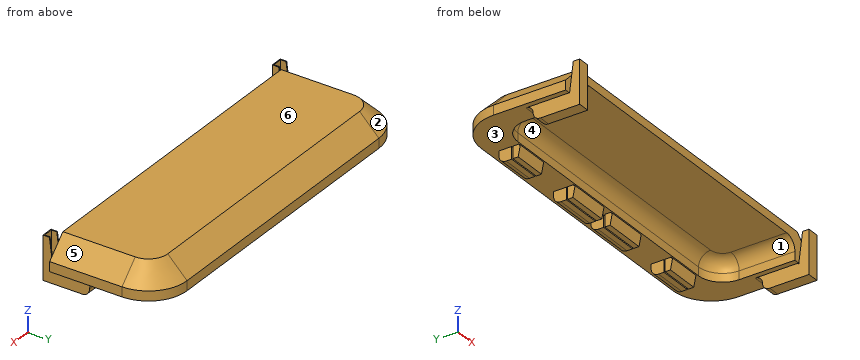
```python
from build123d import *

# Parameters (mm, degrees)
F2_DEPTH      = 12
F3_SIZE       = 8
F0_W          = 14.1
F0_H          = 8.3
F0_W_2        = 40
F4_DEPTH      = 5
F6_DEPTH      = 3
F7_DEPTH      = 20
F7_DEPTH_BACK = 20
F8_START      = 39
F8_DEPTH      = 14.1
F9_START      = -39
F9_DEPTH      = 14.1
F0_W_3        = 4.85
F0_H_2        = 13.3
F10_DEPTH     = 6
F12_DEPTH     = 8.5
F13_W         = 4.85
F13_H         = 5.2
F14_DEPTH     = 6
F15_R         = 2.99999
F16_R         = 5
F17_W         = 5
F17_H         = 8.9
F18_DEPTH     = 5
F20_DEPTH     = 0.8
F21_DEPTH     = 12
F23_DEPTH     = 145.751


# Not quite as in the source:
# - a fillet or chamfer is up to 0.001 mm smaller than in the source, because OpenCascade refuses the exact size


with BuildPart() as f2:
    # F1 (on Top) → F2 (new body)
    with BuildSketch(Plane.XY):
        with BuildLine():
            Line((58, 4), (-58, 4))
            ThreePointArc((-58, 4), (-69.313708499, -0.686291501), (-74, -12))
            Line((-74, -12), (-74, -42))
            Line((-74, -42), (74, -42))
            Line((74, -42), (74, -12))
            ThreePointArc((74, -12), (69.313708499, -0.686291501), (58, 4))
        make_face()
    extrude(amount=F2_DEPTH)

    # F3
    f3_edges = [f2.edges().sort_by_distance(p)[0] for p in [
        (74, -27, 12),
        (0, 4, 12),
        (-74, -27, 12),
    ]]
    chamfer(f3_edges, length=F3_SIZE)

    # F0 (on Top) → F4 (join)
    with BuildSketch(Plane.XY):
        with Locations((-46.05, -4.15)):
            Rectangle(F0_W, F0_H)
        with Locations((0, -4.15)):
            Rectangle(F0_W_2, F0_H)
        with Locations((46.05, -4.15)):
            Rectangle(F0_W, F0_H)
    extrude(amount=-F4_DEPTH)

    # F6 (cut): faces of the model
    f6_faces = [f2.faces().sort_by_distance(p)[0] for p in [
        (0, -8.3, -2.5),
        (46.05, -8.3, -2.5),
        (-46.05, -8.3, -2.5),
    ]]
    extrude(f6_faces, amount=-F6_DEPTH, mode=Mode.SUBTRACT)

    # F5 (on Right) → F7 (join, two sides)
    with BuildSketch(Plane.YZ) as f7_sk:
        Polygon((-5.8, 0), (-8.3, 0), (-8.3, -0.35), (-8.9, -0.55), (-8, -5), (-5.8, -5), align=None)
    extrude(amount=F7_DEPTH)
    extrude(f7_sk.sketch, amount=-F7_DEPTH_BACK)

    # F5 (on Right) → F8 (join)
    with BuildSketch(Plane.YZ.offset(F8_START)):
        Polygon((-5.8, 0), (-8.3, 0), (-8.3, -0.35), (-8.9, -0.55), (-8, -5), (-5.8, -5), align=None)
    extrude(amount=F8_DEPTH)

    # F5 (on Right) → F9 (join)
    with BuildSketch(Plane.YZ.offset(F9_START)):
        Polygon((-5.8, 0), (-8.3, 0), (-8.3, -0.35), (-8.9, -0.55), (-8, -5), (-5.8, -5), align=None)
    extrude(amount=-F9_DEPTH)

    # F0 (on Top) → F10 (join)
    with BuildSketch(Plane.XY):
        with Locations((69.325, -33.65)):
            Rectangle(F0_W_3, F0_H_2)
        with Locations((-69.325, -33.65)):
            Rectangle(F0_W_3, F0_H_2)
    extrude(amount=-F10_DEPTH)

    # F11 (on face) → F12 (cut)
    with BuildSketch(Plane(origin=(0, 0, 0), x_dir=(1, 0, 0), z_dir=(0, 0, -1))):
        with BuildLine():
            Line((64.65, 18.9), (64.65, 42))
            Line((64.65, 42), (-64.65, 42))
            Line((-64.65, 42), (-64.65, 18.9))
            ThreePointArc((-64.65, 18.9), (-61.7210678119, 11.8289321881), (-54.65, 8.9))
            Line((-54.65, 8.9), (54.65, 8.9))
            ThreePointArc((54.65, 8.9), (61.7210678119, 11.8289321881), (64.65, 18.9))
        make_face()
    extrude(amount=-F12_DEPTH, mode=Mode.SUBTRACT)

    # F13 (on face) → F14 (join)
    with BuildSketch(Plane.XZ.offset(40.3)):
        with Locations((69.325, -3.4)):
            Rectangle(F13_W, F13_H)
        with Locations((-69.325, -3.4)):
            Rectangle(F13_W, F13_H)
    extrude(amount=F14_DEPTH)

    # F15 (radius 3 in the source; OpenCascade refuses exactly that, so slightly less here)
    f15_edges = [f2.edges().sort_by_distance(p)[0] for p in [
        (0, 0, -5),
        (-46.05, 0, -5),
        (46.05, 0, -5),
        (-69.325, -27, -6),
        (69.325, -27, -6),
        (69.325, -27, 0),
        (-69.325, -27, 0),
    ]]
    fillet(f15_edges, radius=F15_R)

    # F16
    f16_edges = [f2.edges().sort_by_distance(p)[0] for p in [
        (64.65, -30.45, 8.5),
    ]]
    fillet(f16_edges, radius=F16_R)

    # F17 (on face) → F18 (cut, through all)
    with BuildSketch(Plane(origin=(0, 0, -5), x_dir=(1, 0, 0), z_dir=(0, 0, -1))):
        with Locations((0, 4.45)):
            Rectangle(F17_W, F17_H)
    extrude(amount=-F18_DEPTH, mode=Mode.SUBTRACT)

    # F19 (on face) → F20 (join, through all)
    with BuildSketch(Plane.XY.offset(-0.8)):
        Polygon((71.75, -46.3), (71.75, -40.3), (71.35, -40.3), (71.35, -45.9), (67.3, -45.9), (67.3, -40.3), (66.9, -40.3), (66.9, -46.3), align=None)
        Polygon((-71.35, -40.3), (-71.75, -40.3), (-71.75, -46.3), (-66.9, -46.3), (-66.9, -40.3), (-67.3, -40.3), (-67.3, -45.9), (-71.35, -45.9), align=None)
    extrude(amount=F20_DEPTH)

    # F21 (add, through all): faces of the model
    f21_faces = [f2.faces().sort_by_distance(p)[0] for p in [
        (69.325, -46.2351829498, 0),
        (-71.55, -42.0648170502, 0),
    ]]
    extrude(f21_faces, amount=F21_DEPTH)

    # F22 (on face) → F23 (cut, through all)
    with BuildSketch(Plane.YZ.offset(71.75)):
        Polygon((-42, -0.8), (-42, 12.0000000009), (-43.6490774155, 12), align=None)
    extrude(amount=-F23_DEPTH, mode=Mode.SUBTRACT)


solid = f2.part
```
Geometry check sheet. Reference: the model listing, model coordinates, mm. Face numbers are marked on the shaded views. A direction names the side the tool comes from. Round coordinates to 2 decimals unless told otherwise and drop trailing zeros. Loops run counter-clockwise (first coordinate to the right, second up) from the corner with the lowest first, then second, coordinate; pieces in that order, holes last. Notation, with made-up numbers: M 42,41.5 L 89,41.5 A26 ccw 89,79.5 Z; hole C 42.5,-38.5 d5. An arc over 180 degrees is marked long. Return JSON: item names as keys, results as strings. Group by question number.
(1) Section check B-B, the plane x = -6. Enter the section's corners in (y, z).
(2) Mould release check, pull along X, two halves, no side actions. Record for the marked faces 3, 4, 5 and 6: pulls with the +X half, pulls with the -X half, needs draft (parallel to the pull), parting line crosses it, or undercut.
(3) Set-up check for the marked faces 1 and 2: record each of +Z, -Z, +X, -X, +Y, -Y from which the full face is reachable in a straight line by a thin tool's end or side.
(4) Go/stop test with flat-tipped pins: pin 1 (4 mm diameter, centred on x = -55.5, z = 3, fed in from -Y); pin 2 (5.5 mm diameter, centred on x = -11, z = -1.5, fed in from -Y); pin 3 (2.5 mm diameter, centred on y = -7, z = -3.5, fed in from -X). Record where each tip stops, or that it passes through.
(5) Scan lines: line 1 along X through (y, z) = (-1.5, -1); line 2 along X through (y, z) = (-43.5, 4); line 3 along X through (y, z) = (-41.5, -2.5). Record each from-to range of solid material in increasing order. Write a range as [from, to].
(6) Section check A-A, the plane y = -32. Enter the section's corners in (x, z).
(7) Section check D-D, the plane x = 35.5. Enter the section's corners in (y, z).
(8) Section check C-C, the plane z = 2. Enter the section's corners in (x, y), and give its area (3 significant figures).
Data:
{
 "1": {"outline": "M -42,8.5 L -13.9,8.5 A5 cw -8.9,3.5 L -8.9,0 L -8.3,0 L -8.3,-0.35 L -8.9,-0.55 L -8,-5 L -5.8,-5 L -5.8,0 L -5.3,0 L -5.3,-5 L -3,-5 A3 ccw 0,-2 L 0,0 L 4,0 L 4,4 L -4,12 L -42,12 Z"},
 "2": {"face 3": "undercut", "face 4": "undercut", "face 5": "pulls with the +X half", "face 6": "needs draft"},
 "3": {"face 1": "-Z, -Y", "face 2": "+Z, -X, +Y"},
 "4": {"pin 1": "y = -9.31", "pin 2": "y = -8.9", "pin 3": "x = -53.1"},
 "5": {"line 1": "[-53.1, -39], [-20, -2.5], [2.5, 20], [39, 53.1]", "line 2": "[-71.75, -71.35], [-67.3, -66.9], [66.9, 67.3], [71.35, 71.75]", "line 3": "[-71.75, -66.9], [66.9, 71.75]"},
 "6": {"outline": "M -74,0 L -71.75,0 L -71.75,-6 L -66.9,-6 L -66.9,0 L -64.65,0 L -64.65,3.5 A5 cw -59.65,8.5 L 59.65,8.5 A5 cw 64.65,3.5 L 64.65,0 L 66.9,0 L 66.9,-6 L 71.75,-6 L 71.75,0 L 74,0 L 74,4 L 66,12 L -66,12 L -74,4 Z"},
 "7": {"outline": "M -42,8.5 L -13.9,8.5 A5 cw -8.9,3.5 L -8.9,0 L 4,0 L 4,4 L -4,12 L -42,12 Z"},
 "8": {"outline": "M -74,-42 L -64.65,-42 L -64.65,-18.9 A10 cw -54.65,-8.9 L 54.65,-8.9 A10 cw 64.65,-18.9 L 64.65,-42 L 74,-42 L 74,-12 A16 ccw 58,4 L -58,4 A16 ccw -74,-12 Z; M -71.75,-46.3 L -66.9,-46.3 L -66.9,-42.36 L -67.3,-42.36 L -67.3,-45.9 L -71.35,-45.9 L -71.35,-42.36 L -71.75,-42.36 Z; M 66.9,-46.3 L 71.75,-46.3 L 71.75,-42.36 L 71.35,-42.36 L 71.35,-45.9 L 67.3,-45.9 L 67.3,-42.36 L 66.9,-42.36 Z", "area": "2,470 mm²"}
}
